from build123d import *

# Parameters (mm, degrees)
F1_DEPTH = 63.5
F2_W     = 14.5
F2_H     = 23.934039
F3_DEPTH = 100
F4_R     = 3
F5_DEPTH = 25


with BuildPart() as f1:
    # F0 (on Right) → F1 (new body)
    with BuildSketch(Plane.YZ):
        Polygon((0, 22), (0, 0), (87, 0), (87, 21), (47, 44.5), (43.5, 44.5), align=None)
    extrude(amount=F1_DEPTH)

    # F2 (on face) → F3 (cut)
    with BuildSketch(Plane.XZ):
        with Locations((43.25, 40.958737)):
            Rectangle(F2_W, F2_H)
    extrude(amount=-F3_DEPTH, mode=Mode.SUBTRACT)

    # F4 (on face) → F5 (cut)
    with BuildSketch(Plane.YZ.offset(63.5)):
        with Locations((45.25, 36.5)):
            Circle(F4_R)
    extrude(amount=-F5_DEPTH, mode=Mode.SUBTRACT)


solid = f1.part
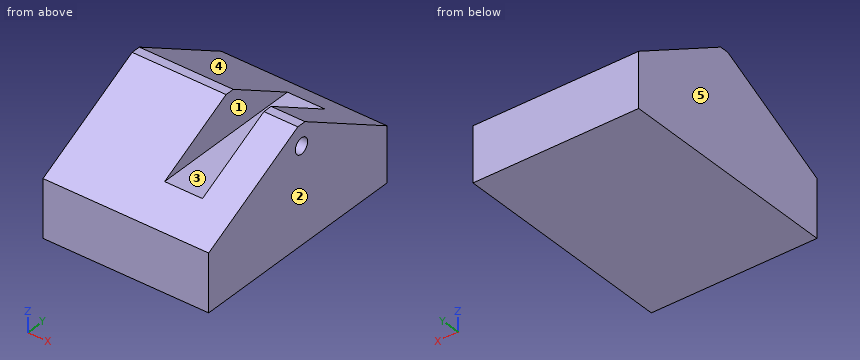
Read the model definition and answer for the solid it produces. Units are mm, in the model's axes. Face numbers are marked on the shaded views. A direction names the side the tool comes from. Round coordinates to 2 decimals unless told otherwise and drop trailing zeros. Write each loop counter-clockwise with the first axis right and the second up, starting at its lowest first coordinate (ties: lowest second). Pieces come first, ordered by that corner, then holes. Notation, with made-up numbers: (84, 74) - (134, 74) arc R12 cw to (134, 88) - close; hole circle Ø2 at (-11.75, -1). An arc over 180 degrees is marked (long way). Use a Markdown table: item, result.
(1) Which of the six approach directions +Z, -Z, +X, -X, +Y, -Y give full straight-line access (tool end or side, diameter ignored) to the marked faces 1 and 2?
Reported:
| item | result |
|---|---|
| face 1 | +Z, +Y, -Y |
| face 2 | +Z, -Z, +X, +Y, -Y |
(2) Straight lines are drawn through the part: line 1 along X through (y, z) = (60.5, 30.5); line 2 along Z through (x, y) = (56.75, 45.25); line 3 along Y through (x, z) = (59, 36). For each, find the intervals that lie inside material, in ascending order. Write a range as [from, to].
Reported:
| item | result |
|---|---|
| line 1 | [0, 36], [50.5, 63.5] |
| line 2 | [0, 33.5], [39.5, 44.5] |
| line 3 | [27.07, 42.29], [48.21, 61.47] |
(3) Each of these flat-tipped pins is pushed along its axis until it touches: pin 1 Ø1.5 at (x, z) = (19, 23) entering from -Y; pin 2 Ø12 at (x, z) = (9.5, 39) entering from -Y; pin 3 Ø5.5 at (y, z) = (45.25, 36.5) entering from +X. Where does it stop, or does it pass through?
Reported:
| item | result |
|---|---|
| pin 1 | y = 0.48 |
| pin 2 | y = 21.27 |
| pin 3 | x = 36 |
(4) The mould has two halves that part along X. Classify the marked faces 3, 4 and 5: released by +X, released by -X, zero draft, split by the parting line, or undercut.
Reported:
| item | result |
|---|---|
| face 3 | undercut |
| face 4 | zero draft |
| face 5 | released by -X |
(5) The part is cut by section C-C (z = 32). Write down the section's boundary in (x, y), then the cut area to 3 significant figures.
Reported:
| item | result |
|---|---|
| outline | (0, 19.33) - (36, 19.33) - (36, 68.28) - (0, 68.28) - close; (50.5, 19.33) - (63.5, 19.33) - (63.5, 68.28) - (50.5, 68.28) - close |
| area | 2,400 mm2 |
(6) The part is cut by section A-A (y = 45.25). Write down the section's boundary in (x, z).
Reported:
| item | result |
|---|---|
| outline | (0, 0) - (63.5, 0) - (63.5, 33.5) - (50.5, 33.5) - (50.5, 28.99) - (36, 28.99) - (36, 44.5) - (0, 44.5) - close; (50.5, 39.5) - (63.5, 39.5) - (63.5, 44.5) - (50.5, 44.5) - close |
(7) The part is cut by section B-B (z = 36.5). Write down the section's boundary in (x, y).
Reported:
| item | result |
|---|---|
| outline | (0, 28.03) - (36, 28.03) - (36, 60.62) - (0, 60.62) - close; (50.5, 28.03) - (63.5, 28.03) - (63.5, 42.25) - (50.5, 42.25) - close; (50.5, 48.25) - (63.5, 48.25) - (63.5, 60.62) - (50.5, 60.62) - close |
(8) The part is cut by section D-D (x = 31.5). Write down the section's boundary in (y, z).
Reported:
| item | result |
|---|---|
| outline | (0, 0) - (87, 0) - (87, 21) - (47, 44.5) - (43.5, 44.5) - (0, 22) - close |
